Verification items for the finished model (mm, model axes). A direction names the side the tool comes from. Coordinates: 2 decimals unless noted, no trailing zeros. Loops run counter-clockwise (first coordinate to the right, second up) from the corner with the lowest first, then second, coordinate; pieces in that order, holes last. Notation, with made-up numbers: (-20, 12.5) -> (24, 12.5) arc R18 ccw to (24, 28.5) -> close; hole circle Ø7 at (53.5, 57.25). An arc over 180 degrees is marked (long way). Write item = value, one per line.
```python
from build123d import *

# Parameters (mm, degrees)
ESQUISSE1_W             = 61.5
ESQUISSE1_H             = 43.75
BOSS_EXTRU_1_DEPTH      = 88
ENL_V_MAT_EXTRU_4_REACH = 90
ESQUISSE3_W             = 53.5
ESQUISSE3_H             = 14.889849441
ESQUISSE6_W             = 57.502648101
ESQUISSE6_H             = 39.75
ENL_V_MAT_EXTRU_5_DEPTH = 82
CONG_4_R                = 2
ESQUISSE7_R             = 1.5
BOSS_EXTRU_2_DEPTH      = 5.2
ESQUISSE8_R             = 1.5
BOSS_EXTRU_3_DEPTH      = 5.2


with BuildPart() as part:
    # Esquisse1 → Boss.-Extru.1 (new body)
    with BuildSketch(Plane.XY):
        with Locations((-0.850502513, 12.751256281)):
            Rectangle(ESQUISSE1_W, ESQUISSE1_H)
    extrude(amount=BOSS_EXTRU_1_DEPTH)

    # Esquisse3 → Enlèv. mat.-Extru.4 (cut, up to next)
    with BuildSketch(Plane.XY.offset(88), mode=Mode.PRIVATE) as enl_v_mat_extru_4_sk1:
        with Locations((-0.850502513, 2.663299217)):
            Rectangle(ESQUISSE3_W, ESQUISSE3_H)
    enl_v_mat_extru_4_tool1 = extrude(enl_v_mat_extru_4_sk1.sketch, amount=-ENL_V_MAT_EXTRU_4_REACH, mode=Mode.PRIVATE) & part.part
    add(enl_v_mat_extru_4_tool1.solids().sort_by_distance((-0.850503, 2.663299, 88))[0], mode=Mode.SUBTRACT)

    # Esquisse6 → Enlèv. mat.-Extru.5 (cut)
    with BuildSketch(Plane(origin=(0, 0, 0), x_dir=(-1, 0, 0), z_dir=(0, 0, -1))):
        with Locations((0.849178462, 12.751256281)):
            Rectangle(ESQUISSE6_W, ESQUISSE6_H)
    extrude(amount=-ENL_V_MAT_EXTRU_5_DEPTH, mode=Mode.SUBTRACT)

    # Congé4
    cong_4_edges = [part.edges().sort_by_distance(p)[0] for p in [
        (29.899497487, 12.751256281, 88),
        (-0.850502513, 34.626256281, 88),
        (-31.600502513, 12.751256281, 88),
        (-31.600502513, 34.626256281, 44),
        (29.899497487, 34.626256281, 44),
        (29.899497487, -9.123743719, 44),
        (-31.600502513, -9.123743719, 44),
        (-0.850502513, -9.123743719, 88),
    ]]
    fillet(cong_4_edges, radius=CONG_4_R)

    # Esquisse7 → Boss.-Extru.2 (add)
    with BuildSketch(Plane(origin=(0, -7.123743719, 0), x_dir=(1, 0, 0), z_dir=(0, 1, 0))):
        with Locations((18.002145588, -9.4)):
            Circle(ESQUISSE7_R)
    extrude(amount=BOSS_EXTRU_2_DEPTH)

    # Esquisse8 → Boss.-Extru.3 (add)
    with BuildSketch(Plane(origin=(0, -7.123743719, 0), x_dir=(1, 0, 0), z_dir=(0, 1, 0))):
        with Locations((-9.850502513, -9.5)):
            Circle(ESQUISSE8_R)
    extrude(amount=BOSS_EXTRU_3_DEPTH)


solid = part.part
```
1) Release check for a two-part mould opening along X. For faces 1 (the face through (-31.601, 12, 42)), 2 (the face through (29.3, 13.03, 87.43)), 3 (the face through (-11.041, -4.56, 10.413)), 4 (the face through (-3, -8, 0)) record: pulls with the +X half, pulls with the -X half, needs draft (parallel to the pull), parting line crosses it, or undercut.
Ans:
face_1 = pulls with the -X half
face_2 = pulls with the +X half
face_3 = undercut
face_4 = needs draft
2) Sectioned sample at B-B, the plane x = 23. Record the cut outline in (y, z), plus the area to 3 significant figures.
Ans:
outline = (-9.12, 0) -> (-7.12, 0) -> (-7.12, 82) -> (-4.78, 82) -> (-4.78, 88) -> (-7.12, 88) arc R2 ccw to (-9.12, 86) -> close; (10.11, 82) -> (32.63, 82) -> (32.63, 0) -> (34.63, 0) -> (34.63, 86) arc R2 ccw to (32.63, 88) -> (10.11, 88) -> close
area = 499 mm2
3) Sectioned sample at D-D, the plane y = 25. Record the cut outline in (x, z).
Ans:
outline = (-31.6, 0) -> (-29.6, 0) -> (-29.6, 82) -> (27.9, 82) -> (27.9, 0) -> (29.9, 0) -> (29.9, 86) arc R2 ccw to (27.9, 88) -> (-29.6, 88) arc R2 ccw to (-31.6, 86) -> close
4) Material ranges on line 1 (X direction, y = -0.5, z = 52); line 2 (Y direction, x = 5.5, z = 48); line 3 (Z direction, x = 17, y = 30), recorded low to high.
Ans:
line_1 = -31.6 to -29.6, 27.9 to 29.9
line_2 = -9.12 to -7.12, 32.63 to 34.63
line_3 = 82 to 88
5) Sectioned sample at C-C, the plane z = 63. Record the cut outline in (x, y), plus the area to 3 significant figures.
Ans:
outline = (-31.6, -7.12) arc R2 ccw to (-29.6, -9.12) -> (27.9, -9.12) arc R2 ccw to (29.9, -7.12) -> (29.9, 32.63) arc R2 ccw to (27.9, 34.63) -> (-29.6, 34.63) arc R2 ccw to (-31.6, 32.63) -> close; hole (-29.6, -7.12) -> (27.9, -7.12) -> (27.9, 32.63) -> (-29.6, 32.63) -> close
area = 401 mm2
6) Depth check by flat-ended pin: pin 1 Ø2 at (x, y) = (-15.5, 27) entering from -Z; pin 2 Ø20 at (x, y) = (-8, 4.5) entering from -Z. Enter the tip coordinate at first touch or a pass-through.
Ans:
pin_1 = 82
pin_2 = 8
7) Sectioned sample at A-A, the plane y = 8.5. Record the cut outline in (x, z).
Ans:
outline = (-31.6, 0) -> (-29.6, 0) -> (-29.6, 82) -> (-27.6, 82) -> (-27.6, 88) -> (-29.6, 88) arc R2 ccw to (-31.6, 86) -> close; (25.9, 82) -> (27.9, 82) -> (27.9, 0) -> (29.9, 0) -> (29.9, 86) arc R2 ccw to (27.9, 88) -> (25.9, 88) -> close
8) Tool access check on faces 5 (the face through (0, 32.626, 40)), 6 (the face through (-1, -9.124, 42)), 7 (the face through (19.433, -4.56, 8.949)), 8 (the face through (29.899, 12, 42)), 9 (the face through (-10, -1.924, 9)). Record the directions out of +Z, -Z, +X, -X, +Y, -Y that give a thin tool (end or side, any length) a straight path to the whole face; none if there is none.
Ans:
face_5 = -Z
face_6 = +Z, -Z, +X, -X, -Y
face_7 = none
face_8 = +Z, -Z, +X, +Y, -Y
face_9 = +Z, -Z
